from build123d import *

# Parameters (mm, degrees)
SKETCH1_W                = 110
SKETCH1_H                = 45
SKETCH1_W_2              = 3
SKETCH1_H_2              = 30
BOSS_EXTRUDE1_DEPTH      = 3
M5_CLEARANCE_HOLE2_D     = 5.5
M5_CLEARANCE_HOLE2_DEPTH = 12.4
M5_CLEARANCE_HOLE2_TIP   = 1.652366702
M5_CLEARANCE_HOLE3_D     = 5.5


with BuildPart() as part:
    # Sketch1 → Boss-Extrude1 (new body)
    with BuildSketch(Plane(origin=(0, 0, 0), x_dir=(1, 0, 0), z_dir=(0, 1, 0))):
        Rectangle(SKETCH1_W, SKETCH1_H)
        Rectangle(SKETCH1_W_2, SKETCH1_H_2, mode=Mode.SUBTRACT)
    extrude(amount=BOSS_EXTRUDE1_DEPTH)

    # M5 Clearance Hole2
    with Locations(Plane(origin=(0, 3, 0), x_dir=(1, 0, 0), z_dir=(0, 1, 0))):
        with Locations((50, 15), (-50, -15), (-50, 15), (50, -15)):
            Hole(M5_CLEARANCE_HOLE2_D / 2, depth=M5_CLEARANCE_HOLE2_DEPTH)
            with Locations((0, 0, -(M5_CLEARANCE_HOLE2_DEPTH + M5_CLEARANCE_HOLE2_TIP / 2))):  # 118° drill point
                Cone(0, M5_CLEARANCE_HOLE2_D / 2, M5_CLEARANCE_HOLE2_TIP, mode=Mode.SUBTRACT)

    # M5 Clearance Hole3 (through all)
    with Locations(Plane(origin=(0, 3, 0), x_dir=(1, 0, 0), z_dir=(0, 1, 0))):
        with Locations((-25.4, -12.7), (25.4, 12.7), (-25.4, 12.7), (25.4, -12.7)):
            Hole(M5_CLEARANCE_HOLE3_D / 2)


solid = part.part
Read the model definition and answer for the solid it produces. Units are mm, in the model's axes. A direction names the side the tool comes from. Coordinates: 2 decimals unless noted, no trailing zeros. Loops run counter-clockwise (first coordinate to the right, second up) from the corner with the lowest first, then second, coordinate; pieces in that order, holes last. Notation, with made-up numbers: (5.25, 8.5) -> (42.25, 8.5) arc R17 cw to (42.25, 28.5) -> close; hole circle Ø2 at (6, 4). An arc over 180 degrees is marked (long way). Write item = value, one per line. Start each with the question number.
1) Given P1, Ø3, axis at x = 38.5, z = 11.5, coming from the -Y side, flat-ended and moving along its own axis, determine where the tip first touches the part or whether it passes through.
2) Find the intervals of material crossed by L1, parallel to Z at x = 50, y = 0.7; L2, parallel to Z at x = 25.4, y = 1.4; L3, parallel to X at y = 1.1, z = 12, in increasing order. Write a range as from..to.
3) For faces 5 (the face through (55, 1, 0)), 6 (the face through (0, 1, -15)), determine the directions among +Z, -Z, +X, -X, +Y, -Y from which every point of the face is accessible in a straight line to the end or side of a thin tool.
4) The mould has two halves that part along Z. Classify faces 1 (the face through (-1, 1, -22.5)), 2 (the face through (-23.218, 1.479, 14.373)), 3 (the face through (-55, 1, 0)), 4 (the face through (-1, 1, 22.5)): pulls with the +Z half, pulls with the -Z half, needs draft (parallel to the pull), parting line crosses it, or undercut.
5) The part is cut by section A-A, the plane x = -25.4. Determine the outline of the cut face in (y, z), plus the area to 3 significant figures.
6) The part is cut by section C-C, the plane z = -3. Determine the outline of the cut face in (x, y).
7) The part is cut by section B-B, the plane y = 1.5. State how many separate pieces and enclosed holes the cut face has, plus the area to 3 significant figures.
Result:
q1.P1 = 0
q2.L1 = -22.5..-17.75, -12.25..12.25, 17.75..22.5
q2.L2 = -22.5..-15.45, -9.95..9.95, 15.45..22.5
q2.L3 = -55..-28.06, -22.74..-1.5, 1.5..22.74, 28.06..55
q3.face_5 = +Z, -Z, +X, +Y, -Y
q3.face_6 = +Y, -Y
q4.face_1 = pulls with the -Z half
q4.face_2 = undercut
q4.face_3 = needs draft
q4.face_4 = pulls with the +Z half
q5.outline = (0, -22.5) -> (3, -22.5) -> (3, -15.45) -> (0, -15.45) -> close; (0, -9.95) -> (3, -9.95) -> (3, 9.95) -> (0, 9.95) -> close; (0, 15.45) -> (3, 15.45) -> (3, 22.5) -> (0, 22.5) -> close
q5.area = 102 mm²
q6.outline = (-55, 0) -> (-1.5, 0) -> (-1.5, 3) -> (-55, 3) -> close; (1.5, 0) -> (55, 0) -> (55, 3) -> (1.5, 3) -> close
q7.separate_pieces = 1
q7.enclosed_holes = 9
q7.area = 4,670 mm²
